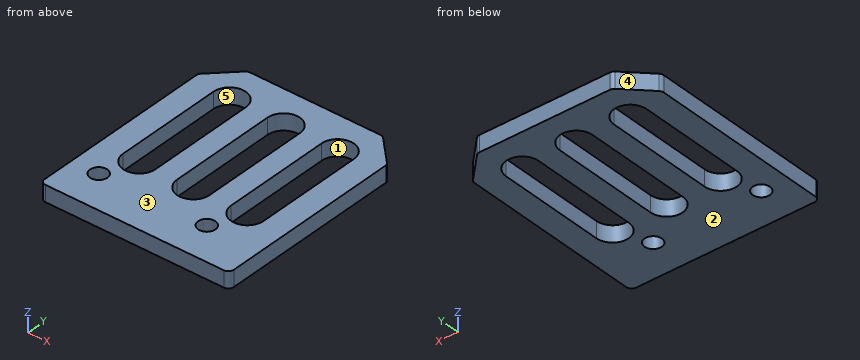
```python
from build123d import *

# Parameters (mm, degrees)
SKETCH_1_W          = 35
SKETCH_1_H          = 40
EXTRUDE_1_DEPTH     = 3
CHAMFER_1_SIZE      = 5
FILLET_1_R          = 1
SKETCH_2_R          = 1.6
CUT_EXTRUDE_1_DEPTH = 4
CUT_EXTRUDE_2_DEPTH = 4


with BuildPart() as part:
    # 草图1 → 凸台-拉伸1 (new body)
    with BuildSketch(Plane.XY):
        Rectangle(SKETCH_1_W, SKETCH_1_H)
    extrude(amount=EXTRUDE_1_DEPTH)

    # 倒角1
    chamfer_1_edges = [part.edges().sort_by_distance(p)[0] for p in [
        (-17.5, 20, 1.5),
        (17.5, 20, 1.5),
    ]]
    chamfer(chamfer_1_edges, length=CHAMFER_1_SIZE)

    # 圆角1
    fillet_1_edges = [part.edges().sort_by_distance(p)[0] for p in [
        (-17.5, 15, 1.5),
        (12.5, 20, 1.5),
        (-12.5, 20, 1.5),
        (17.5, 15, 1.5),
        (17.5, -20, 1.5),
        (-17.5, -20, 1.5),
    ]]
    fillet(fillet_1_edges, radius=FILLET_1_R)

    # 草图2 → 切除-拉伸1 (cut, through all)
    with BuildSketch(Plane.XY.offset(3)):
        with Locations((-12.5, -13)):
            Circle(SKETCH_2_R)
        with Locations((7.5, -13)):
            Circle(SKETCH_2_R)
    extrude(amount=-CUT_EXTRUDE_1_DEPTH, mode=Mode.SUBTRACT)

    # 草图3 → 切除-拉伸2 (cut, through all)
    with BuildSketch(Plane.XY.offset(3)):
        with BuildLine():
            Line((3, 13), (3, -7))
            ThreePointArc((3, -7), (0, -10), (-3, -7))
            Line((-3, -7), (-3, 13))
            ThreePointArc((-3, 13), (0, 16), (3, 13))
        make_face()
        with BuildLine():
            Line((-7, 13), (-7, -7))
            ThreePointArc((-7, -7), (-10, -10), (-13, -7))
            Line((-13, -7), (-13, 13))
            ThreePointArc((-13, 13), (-10, 16), (-7, 13))
        make_face()
        with BuildLine():
            Line((13, 13), (13, -7))
            ThreePointArc((13, -7), (10, -10), (7, -7))
            Line((7, -7), (7, 13))
            ThreePointArc((7, 13), (10, 16), (13, 13))
        make_face()
    extrude(amount=-CUT_EXTRUDE_2_DEPTH, mode=Mode.SUBTRACT)


solid = part.part
```
The model under review builds one solid part; all positions refer to its coordinate system, in mm. Face numbers are marked on the shaded views. A direction names the side the tool comes from. Give positions to 0.01 mm unless a question says otherwise; leave off trailing zeros. Write each loop counter-clockwise with the first axis right and the second up, starting at its lowest first coordinate (ties: lowest second). Pieces come first, ordered by that corner, then holes. Notation, with made-up numbers: (62.25, -17) - (94.25, -17) arc R18 cw to (94.25, -10) - close; hole circle Ø5 at (50, 83.25). An arc over 180 degrees is marked (long way). Answer in a Markdown table with one row per item. Add a question column.
1. We need section A-A on x = 10. Write out the cut boundary in (y, z), then the cut area to 3 significant figures.
2. We need section B-B on y = -13. Write out the cut boundary in (x, z).
3. Tool access review of the marked faces 1 and 2: name each direction out of +Z, -Z, +X, -X, +Y, -Y from which nothing blocks a thin tool from reaching the whole face with its end or side.
4. Wall thickness on line 1 along X through (y, z) = (5, 0.75); line 2 along Y through (x, z) = (-12.5, 0.75); line 3 along Y through (x, z) = (15, 0.55): over which ranges is each line inside the solid? List them lowest first. Write a range as [from, to].
5. We need section C-C on z = 0.65. Write out the cut boundary in (x, y).
6. We need section D-D on y = 5.5. Write out the cut boundary in (x, z).
7. Draft analysis for pull direction X (two halves, no side actions). For the marked faces 3, 4 and 5, state which applies: +X half, -X half, draft (parallel to the pull), parting line (faces both ways), or undercut.
Ans:
| question | item | result |
|---|---|---|
| 1 | outline | (-20, 0) - (-10, 0) - (-10, 3) - (-20, 3) - close; (16, 0) - (20, 0) - (20, 3) - (16, 3) - close |
| 1 | area | 42.0 mm^2 |
| 2 | outline | (-17.5, 0) - (-14.1, 0) - (-14.1, 3) - (-17.5, 3) - close; (-10.9, 0) - (5.9, 0) - (5.9, 3) - (-10.9, 3) - close; (9.1, 0) - (17.5, 0) - (17.5, 3) - (9.1, 3) - close |
| 3 | face 1 | +Z, -Z |
| 3 | face 2 | -Z, +X, -X, +Y, -Y |
| 4 | line 1 | x = [-17.5, -13], [-7, -3], [3, 7], [13, 17.5] |
| 4 | line 2 | y = [-20, -14.6], [-11.4, -8.66], [14.66, 19.91] |
| 4 | line 3 | y = [-20, 17.5] |
| 5 | outline | (-17.5, -19) arc R1 ccw to (-16.5, -20) - (16.5, -20) arc R1 ccw to (17.5, -19) - (17.5, 14.59) arc R1 ccw to (17.21, 15.29) - (12.79, 19.71) arc R1 ccw to (12.09, 20) - (-12.09, 20) arc R1 ccw to (-12.79, 19.71) - (-17.21, 15.29) arc R1 ccw to (-17.5, 14.59) - close; hole circle Ø3.2 at (-12.5, -13); hole (-13, -7) arc R3 ccw to (-7, -7) - (-7, 13) arc R3 ccw to (-13, 13) - close; hole (-3, -7) arc R3 ccw to (3, -7) - (3, 13) arc R3 ccw to (-3, 13) - close; hole circle Ø3.2 at (7.5, -13); hole (7, -7) arc R3 ccw to (13, -7) - (13, 13) arc R3 ccw to (7, 13) - close |
| 6 | outline | (-17.5, 0) - (-13, 0) - (-13, 3) - (-17.5, 3) - close; (-7, 0) - (-3, 0) - (-3, 3) - (-7, 3) - close; (3, 0) - (7, 0) - (7, 3) - (3, 3) - close; (13, 0) - (17.5, 0) - (17.5, 3) - (13, 3) - close |
| 7 | face 3 | draft |
| 7 | face 4 | -X half |
| 7 | face 5 | undercut |
